Source: CAD feature listing. Evaluate the final solid. Frame: model axes, mm. A direction names the side the tool comes from. Coordinates: 2 decimals unless noted, no trailing zeros. Order: outer loops, then holes, each group sorted by start corner. A loop starts at its lowest first (then second) coordinate and runs counter-clockwise, first axis right, second up.
Item 1: Section A-A on y = 12.5. Return the cut outline in (x, z), then the cut area to 3 significant figures.
Item 2: Reachability of faces 1 (the flat face through (-43, -1, 23)), 2 (the flat face through (-43, 13, -9)), 3 (the flat face through (41, 10, 27)) from +Z, -Z, +X, -X, +Y, -Y: full face, straight path, thin tool, end or side. Return the list, or none.
Item 3: Ray query, line 1 (X direction, y = 15.25, z = 25); line 2 (Y direction, x = -9, z = 11.5). Return the intervals inside material, ascending.
Item 4: Mould query, pull axis Z, two halves, no side actions, for faces 4 (the flat face through (-10, 20, 10)), 5 (the flat face through (-24, -1, 43)), 6 (the cylindrical face through (-43.528, 5.295, 23.706)), 7 (the flat face through (-41, 10, 1)). Classes: released by +Z, released by -Z, zero draft, split by the parting line, or undercut.
Item 5: Section B-B on z = 32.5. Return the cut outline in (x, y).
Item 6: Contact query for flat-ended pins moving along their axis: P1, Ø6, axis at x = -31, y = 6.5, coming from the +Z side; P2, Ø1, axis at x = -4, z = -20, coming from the -Y side; P3, Ø2, axis at x = 32.5, y = 3.5, coming from the -Z side. Output: stop coordinate, or through.
Item 7: Section D-D on y = 5.75. Return the cut outline in (x, z).
Item 8: Section C-C on x = -24. Return the cut outline in (y, z).
from build123d import *

# Parameters (mm, degrees)
BOSS_EXTRUDE1_DEPTH = 20
SKETCH2_W           = 86
SKETCH2_H           = 86
BOSS_EXTRUDE2_DEPTH = 2
CUT_EXTRUDE1_DEPTH  = 20
SKETCH4_W           = 2
SKETCH4_H           = 40
SKETCH4_W_2         = 40
SKETCH4_H_2         = 2
BOSS_EXTRUDE4_DEPTH = 2.5
FILLET1_R           = 10


with BuildPart() as part:
    # Sketch1 → Boss-Extrude1 (new body)
    with BuildSketch(Plane(origin=(0, 0, 0), x_dir=(1, 0, 0), z_dir=(0, 1, 0))):
        Polygon((-43, 43), (-43, -43), (14.982756057, 14.982756057), (-13.034487885, 43), align=None)
        Polygon((14.982756057, 14.982756057), (-43, -43), (43, -43), (43, -13.034487885), align=None)
    extrude(amount=BOSS_EXTRUDE1_DEPTH)

    # Sketch2 → Boss-Extrude2 (add)
    with BuildSketch(Plane(origin=(0, 20, 0), x_dir=(1, 0, 0), z_dir=(0, 1, 0))):
        Rectangle(SKETCH2_W, SKETCH2_H)
    extrude(amount=BOSS_EXTRUDE2_DEPTH)

    # Sketch3 → Cut-Extrude1 (cut)
    with BuildSketch(Plane.XZ):
        Polygon((-13.86291501, -41), (41, 13.86291501), (41, 41), (-41, 41), (-41, -41), align=None)
    extrude(amount=-CUT_EXTRUDE1_DEPTH, mode=Mode.SUBTRACT)

    # Sketch4 → Boss-Extrude4 (add, symmetric)
    with BuildSketch(Plane.XZ):
        with Locations((-44, 23)):
            Rectangle(SKETCH4_W, SKETCH4_H)
        with Locations((-25, 44)):
            Rectangle(SKETCH4_W_2, SKETCH4_H_2)
    extrude(amount=BOSS_EXTRUDE4_DEPTH, both=True)

    # Fillet1
    # the kernel refuses this fillet: 10 mm, written as the material it adds along each edge
    with BuildSketch(Plane(origin=(-43, 2.5, 3), x_dir=(0, 1, 0), z_dir=(0, 0, 1))) as fillet1_piece_1:
        with BuildLine():
            CenterArc((6, 10), FILLET1_R, 233.130102354, 36.869897646)
            Line((0, 2), (-0.12, 1.84))
            ThreePointArc((-0.12, 1.84), (-0.2, 1), (-0.2, 0))
            Line((-0.2, 0), (0, -0.2))
            Line((0, -0.2), (6, -0.2))
            Line((6, -0.2), (6, 0))
        make_face()
    extrude(amount=40)
    with BuildSketch(Plane(origin=(-5, 2.5, 43), x_dir=(0, 0, 1), z_dir=(-1, 0, 0))) as fillet1_piece_2:
        with BuildLine():
            CenterArc((10, 6), FILLET1_R, 180, 36.869897646)
            Line((0, 6), (-0.2, 6))
            Line((-0.2, 6), (-0.2, 0))
            Line((-0.2, 0), (0, -0.2))
            ThreePointArc((0, -0.2), (1, -0.2), (1.84, -0.12))
            Line((1.84, -0.12), (2, 0))
        make_face()
    extrude(amount=38)
    with BuildSketch(Plane(origin=(-43, 2.5, 3), x_dir=(0, 1, 0), z_dir=(0, 0, 1))) as fillet1_piece_3a_section:
        with BuildLine():
            CenterArc((6, 10), FILLET1_R, 233.130102354, 36.869897646)
            Line((0, 2), (-0.12, 1.84))
            ThreePointArc((-0.12, 1.84), (-0.2, 1), (-0.2, 0))
            Line((-0.2, 0), (0, -0.2))
            Line((0, -0.2), (6, -0.2))
            Line((6, -0.2), (6, 0))
        make_face()
    fillet1_piece_3a = extrude(amount=55, mode=Mode.PRIVATE)
    fillet1_piece_3a = split(fillet1_piece_3a, bisect_by=Plane(origin=(-43.452376795, 4.199345627, 43), z_dir=(0, 0, 1)), keep=Keep.TOP, mode=Mode.PRIVATE)
    fillet1_piece_3a = split(fillet1_piece_3a, bisect_by=Plane(origin=(-43.452376795, 4.199345627, 45), z_dir=(0, 0, -1)), keep=Keep.TOP, mode=Mode.PRIVATE)
    with BuildSketch(Plane(origin=(-5, 2.5, 43), x_dir=(0, 0, 1), z_dir=(-1, 0, 0))) as fillet1_piece_3b_section:
        with BuildLine():
            CenterArc((10, 6), FILLET1_R, 180, 36.869897646)
            Line((0, 6), (-0.2, 6))
            Line((-0.2, 6), (-0.2, 0))
            Line((-0.2, 0), (0, -0.2))
            ThreePointArc((0, -0.2), (1, -0.2), (1.84, -0.12))
            Line((1.84, -0.12), (2, 0))
        make_face()
    fillet1_piece_3b = extrude(amount=53, mode=Mode.PRIVATE)
    fillet1_piece_3b = split(fillet1_piece_3b, bisect_by=Plane(origin=(-43, 4.199345627, 43.452376795), z_dir=(-1, 0, 0)), keep=Keep.TOP, mode=Mode.PRIVATE)
    fillet1_piece_3b = split(fillet1_piece_3b, bisect_by=Plane(origin=(-45, 4.199345627, 43.452376795), z_dir=(1, 0, 0)), keep=Keep.TOP, mode=Mode.PRIVATE)
    fillet1_piece_3 = fillet1_piece_3a & fillet1_piece_3b
    add(fillet1_piece_3)


solid = part.part
Answer list:
1. outline: (-43, -43) - (-13.03, -43) - (43, 13.03) - (43, 43) - (-43, 43) - close; hole (-41, -41) - (-13.86, -41) - (41, 13.86) - (41, 41) - (-41, 41) - close
1. area: 607 mm2
2. face 1: -Z, +X, -Y
2. face 2: -Z, -X, +Y
2. face 3: -Y
3. line 1: x = -43 to -41, 41 to 43
3. line 2: y = 20 to 22
4. face 4: undercut
4. face 5: released by -Z
4. face 6: zero draft
4. face 7: undercut
5. outline: (-45, -2.5) - (-43, -2.5) - (-43, 0) - (-41, 0) - (-41, 20) - (41, 20) - (41, 0) - (43, 0) - (43, 22) - (-43, 22) - (-43, 8.5) arc R10 cw to (-45, 2.5) - close
6. P1: stops at z = 44.34
6. P2: stops at y = 20
6. P3: stops at z = 1.53
7. outline: (-43.39, 3) - (-43, 3) - (-43, -43) - (-13.03, -43) - (43, 13.03) - (43, 43) - (-5, 43) - (-5, 43.39) - (-43.39, 43.39) - close; hole (-41, -41) - (-13.86, -41) - (41, 13.86) - (41, 41) - (-41, 41) - close
8. outline: (-2.5, 43) - (0, 43) - (0, 41) - (20, 41) - (20, -41) - (0, -41) - (0, -43) - (22, -43) - (22, 43) - (8.5, 43) arc R10 cw to (2.5, 45) - (-2.5, 45) - close
